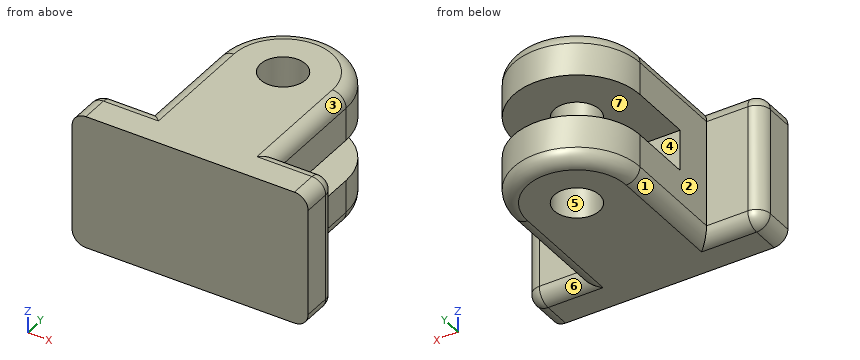
from build123d import *

# Parameters (mm, degrees)
SKETCH1_R           = 1.6375
BOSS_EXTRUDE1_DEPTH = 4.875
SKETCH3_R           = 1.6375
CUT_EXTRUDE1_DEPTH  = 1.5
FILLET1_R           = 1


with BuildPart() as part:
    # Sketch1 → Boss-Extrude1 (new body, symmetric)
    with BuildSketch(Plane.XY):
        with BuildLine():
            Line((-4.5875, 0), (-4.5875, -7.5875))
            Line((-4.5875, -7.5875), (-8.5875, -7.5875))
            Line((-8.5875, -7.5875), (-8.5875, -10.5875))
            Line((-8.5875, -10.5875), (8.5875, -10.5875))
            Line((8.5875, -10.5875), (8.5875, -7.5875))
            Line((8.5875, -7.5875), (4.5875, -7.5875))
            Line((4.5875, -7.5875), (4.5875, 0))
            ThreePointArc((4.5875, 0), (0, 4.5875), (-4.5875, 0))
        make_face()
        Circle(SKETCH1_R, mode=Mode.SUBTRACT)
    extrude(amount=BOSS_EXTRUDE1_DEPTH, both=True)

    # Sketch3 → Cut-Extrude1 (cut, symmetric)
    with BuildSketch(Plane.XY):
        with BuildLine():
            Line((-4.5875, 0), (-4.5875, -4.5875))
            Line((-4.5875, -4.5875), (4.5875, -4.5875))
            Line((4.5875, -4.5875), (4.5875, 0))
            ThreePointArc((4.5875, 0), (0, 4.5875), (-4.5875, 0))
        make_face()
        Circle(SKETCH3_R, mode=Mode.SUBTRACT)
    extrude(amount=CUT_EXTRUDE1_DEPTH, both=True, mode=Mode.SUBTRACT)

    # Fillet1
    fillet1_edges = [part.edges().sort_by_distance(p)[0] for p in [
        (-6.5875, -7.5875, 4.875),
        (-4.5875, -3.79375, -4.875),
        (0, 4.5875, -4.875),
        (-8.5875, -9.0875, 4.875),
        (8.5875, -7.5875, 0),
        (-8.5875, -7.5875, 0),
        (8.5875, -9.0875, 4.875),
        (6.5875, -7.5875, 4.875),
        (4.5875, -3.79375, 4.875),
        (0, 4.5875, 4.875),
        (-4.5875, -3.79375, 4.875),
        (4.5875, -3.79375, -4.875),
        (6.5875, -7.5875, -4.875),
        (8.5875, -9.0875, -4.875),
        (-8.5875, -9.0875, -4.875),
        (-6.5875, -7.5875, -4.875),
    ]]
    fillet(fillet1_edges, radius=FILLET1_R)


solid = part.part
Work out the finished part from the listing and answer in its coordinate system (mm). Face numbers are marked on the shaded views. A direction names the side the tool comes from. Give positions to 0.01 mm unless a question says otherwise; leave off trailing zeros. Loops run counter-clockwise (first coordinate to the right, second up) from the corner with the lowest first, then second, coordinate; pieces in that order, holes last. Notation, with made-up numbers: (14.5, 36) - (61.5, 36) arc R27 cw to (61.5, 53) - close; hole circle Ø4 at (16.5, -3). An arc over 180 degrees is marked (long way). Answer in a Markdown table with one row per item. Add a question column.
Q1. Each of these flat-tipped pins is pushed along its axis until it touches: P1, Ø4, axis at x = -1, y = -0.5, coming from the +Z side (3 decimals); P2, Ø1.5, axis at x = -6, z = -0.5, coming from the +Y side; P3, Ø0.9, axis at x = 1.5, z = 0.5, coming from the +Y side; P4, Ø5, axis at y = -2.5, z = -1, coming from the +X side. Where does it stop, or does it pass through?
Q2. The part is cut by section B-B (z = 3). Determine the outline of the cut face in (x, y) (1 decimal), and give its area (3 significant figures).
Q3. Consider line 1 along Z through (x, y) = (-2, -2.25) (3 decimals); line 2 along Y through (x, z) = (0, 3); line 3 along Z through (x, y) = (4, -1.75). Determine where each line is inside the solid, lowest interval first.
Q4. A tool of negligible diameter and unlimited length cuts with its end or side. For the marked faces 1, 2, 3 and 4, from which of +Z, -Z, +X, -X, +Y, -Y can it reach the whole face along a straight path? Write none if from no direction.
Q5. The part is cut by section D-D (z = -0.5). Determine the outline of the cut face in (x, y), and give its area (3 significant figures).
Q6. Determine the mould class of the marked faces 5, 6 and 7 for opening direction Y: released by +Y, released by -Y, zero draft, split by the parting line, or undercut.
Q7. The part is cut by section C-C (x = 0). Determine the outline of the cut face in (y, z) (1 decimal).
Q8. The part is cut by section A-A (y = -3.25). Determine the outline of the cut face in (x, z) (1 decimal).
Solution:
| question | item | result |
|---|---|---|
| 1 | P1 | stops at z = 4.875 |
| 1 | P2 | stops at y = -7.59 |
| 1 | P3 | stops at y = -4.59 |
| 1 | P4 | stops at x = 4.59 |
| 2 | outline | (-8.6, -10.6) - (8.6, -10.6) - (8.6, -8.6) arc R1 ccw to (7.6, -7.6) - (4.6, -7.6) - (4.6, 0) arc R4.6 ccw to (-4.6, 0) - (-4.6, -7.6) - (-7.6, -7.6) arc R1 ccw to (-8.6, -8.6) - close; hole circle Ø3.3 at (0, 0) |
| 2 | area | 145 mm² |
| 3 | line 1 | z = -4.875 to -1.5, 1.5 to 4.875 |
| 3 | line 2 | y = -10.59 to -1.64, 1.64 to 4.59 |
| 3 | line 3 | z = -4.79 to -1.5, 1.5 to 4.79 |
| 4 | face 1 | -Z, -X, +Y |
| 4 | face 2 | +Z, -Z, -X, +Y |
| 4 | face 3 | +Z, +X, +Y |
| 4 | face 4 | +X, -X, +Y |
| 5 | outline | (-8.59, -10.59) - (8.59, -10.59) - (8.59, -8.59) arc R1 ccw to (7.59, -7.59) - (4.59, -7.59) - (4.59, -4.59) - (-4.59, -4.59) - (-4.59, -7.59) - (-7.59, -7.59) arc R1 ccw to (-8.59, -8.59) - close |
| 5 | area | 78.6 mm² |
| 6 | face 5 | undercut |
| 6 | face 6 | released by +Y |
| 6 | face 7 | zero draft |
| 7 | outline | (-10.6, -4.9) - (-1.6, -4.9) - (-1.6, -1.5) - (-4.6, -1.5) - (-4.6, 1.5) - (-1.6, 1.5) - (-1.6, 4.9) - (-10.6, 4.9) - close; (1.6, -4.9) - (3.6, -4.9) arc R1 ccw to (4.6, -3.9) - (4.6, -1.5) - (1.6, -1.5) - close; (1.6, 1.5) - (4.6, 1.5) - (4.6, 3.9) arc R1 ccw to (3.6, 4.9) - (1.6, 4.9) - close |
| 8 | outline | (-4.6, -3.9) arc R1 ccw to (-3.6, -4.9) - (3.6, -4.9) arc R1 ccw to (4.6, -3.9) - (4.6, -1.5) - (-4.6, -1.5) - close; (-4.6, 1.5) - (4.6, 1.5) - (4.6, 3.9) arc R1 ccw to (3.6, 4.9) - (-3.6, 4.9) arc R1 ccw to (-4.6, 3.9) - close |
